Read the model definition and answer for the solid it produces. Units are mm, in the model's axes. A direction names the side the tool comes from. Coordinates: 2 decimals unless noted, no trailing zeros. Order: outer loops, then holes, each group sorted by start corner. A loop starts at its lowest first (then second) coordinate and runs counter-clockwise, first axis right, second up. Notation, with made-up numbers: M -19,79.5 L -15,79.5 A24 ccw -15,108.5 Z; hole C 15,28 d9. An arc over 180 degrees is marked long. Use a Markdown table: item, result. Add a question column.
1) Find the intervals of material crossed by probe 1 along X at (y, z) = (17, -4); probe 2 along X at (y, z) = (4.25, 34.5); probe 3 along Z at (x, y) = (10.5, 22), in increasing order. Write a range as [from, to].
2) Each of these flat-tipped pins is pushed along its axis until it touches: pin 1 Ø6.5 at (y, z) = (9.5, -5) entering from -X; pin 2 Ø4 at (y, z) = (12, 5.5) entering from +X; pin 3 Ø7 at (y, z) = (11, 37.5) entering from -X. Where does it stop, or does it pass through?
3) Find section B-B on z = -4. Write down the section's boundary in (x, y), plus the area to 3 significant figures.
4) Find section D-D on x = 15. Write down the section's boundary in (y, z), plus the area to 3 significant figures.
5) Find section C-C on y = 8.75. Write down the section's boundary in (x, z).
6) The mould has two halves that part along Z. Classify faces 1 (the face through (45, 10, -8)), 2 (the face through (44, 10, 49.85)), 3 (the face through (42.548, 19.57, 45.416)): released by +Z, released by -Z, zero draft, split by the parting line, or undercut.
7) Find section A-A on y = 20.5. Write down the section's boundary in (x, z), plus the area to 3 significant figures.
8) For faces 4 (the face through (54, 10, 32.85)), 5 (the face through (45, 14.5, -4)), 6 (the face through (20, 10, 41.85)), 7 (the face through (40.5, 10, -4)), determine the directions among +Z, -Z, +X, -X, +Y, -Y from which every point of the face is accessible in a straight line to the end or side of a thin tool.
from build123d import *

# Parameters (mm, degrees)
BOSS_EXTRUDE1_DEPTH  = 24.5
SKETCH2_W            = 103
SKETCH2_H            = 41.85
BOSS_EXTRUDE2_DEPTH  = 5
SKETCH3_W            = 46.5
SKETCH3_H            = 27.85
CUT_EXTRUDE1_DEPTH   = 26
SKETCH7_W            = 8
SKETCH7_H            = 3
BOSS_EXTRUDE3_DEPTH  = 8
SKETCH8_R            = 2.5
CUT_EXTRUDE2_DEPTH   = 8
SKETCH9_W            = 8
SKETCH9_H            = 3
BOSS_EXTRUDE4_DEPTH  = 8
SKETCH10_R           = 2.5
CUT_EXTRUDE3_DEPTH   = 8
SKETCH12_W           = 11.5
SKETCH12_H           = 5
CUT_EXTRUDE4_DEPTH   = 8
SKETCH14_W           = 8
SKETCH14_H           = 3
BOSS_EXTRUDE5_DEPTH  = 8
SKETCH15_R           = 2.5
CUT_EXTRUDE5_DEPTH   = 8
SKETCH16_W           = 8
SKETCH16_H           = 29.5
BOSS_EXTRUDE6_DEPTH  = 8
SKETCH17_W           = 14
SKETCH17_H           = 29.5
BOSS_EXTRUDE7_DEPTH  = 8
SKETCH18_R           = 2
CUT_EXTRUDE6_DEPTH   = 10
SKETCH19_W           = 8
SKETCH19_H           = 29.5
BOSS_EXTRUDE8_DEPTH  = 8
SKETCH20_W           = 13
SKETCH20_H           = 13
BOSS_EXTRUDE9_DEPTH  = 88
CUT_EXTRUDE8_DEPTH   = 48
SKETCH23_R           = 2.5
CUT_EXTRUDE9_DEPTH   = 10
SKETCH25_W           = 8
SKETCH25_H           = 3
CUT_EXTRUDE10_DEPTH  = 8
SKETCH27_W           = 8
SKETCH27_H           = 29.5
BOSS_EXTRUDE11_DEPTH = 8
SKETCH28_R           = 2.5
CUT_EXTRUDE12_DEPTH  = 15
SKETCH29_W           = 13
SKETCH29_H           = 13
CUT_EXTRUDE13_DEPTH  = 88
SKETCH30_W           = 14
SKETCH30_H           = 8
CUT_EXTRUDE14_DEPTH  = 147


with BuildPart() as part:
    # Sketch1 → Boss-Extrude1 (new body)
    with BuildSketch(Plane(origin=(0, 0, 0), x_dir=(1, 0, 0), z_dir=(0, 1, 0))):
        Polygon((0, 0), (51.5, 0), (51.5, -5), (5, -5), (5, -36.85), (51.5, -36.85), (51.5, -32.85), (56.5, -32.85), (56.5, -41.85), (0, -41.85), align=None)
    extrude(amount=BOSS_EXTRUDE1_DEPTH)

    # Sketch2 → Boss-Extrude2 (add)
    with BuildSketch(Plane.XZ):
        with Locations((51.5, 20.925)):
            Rectangle(SKETCH2_W, SKETCH2_H)
    extrude(amount=BOSS_EXTRUDE2_DEPTH)

    # Sketch3 → Cut-Extrude1 (cut)
    with BuildSketch(Plane(origin=(0, 0, 0), x_dir=(1, 0, 0), z_dir=(0, 1, 0))):
        with Locations((74.75, -18.925)):
            Rectangle(SKETCH3_W, SKETCH3_H)
    extrude(amount=-CUT_EXTRUDE1_DEPTH, mode=Mode.SUBTRACT)

    # Sketch7 → Boss-Extrude3 (add)
    with BuildSketch(Plane.XY.offset(41.85)):
        with Locations((4, -3.5)):
            Rectangle(SKETCH7_W, SKETCH7_H)
    extrude(amount=BOSS_EXTRUDE3_DEPTH)

    # Sketch8 → Cut-Extrude2 (cut)
    with BuildSketch(Plane(origin=(0, -2, 0), x_dir=(1, 0, 0), z_dir=(0, 1, 0))):
        with Locations(Location((4, -45.85, 0), (0, 0, 270))):
            Circle(SKETCH8_R)
    extrude(amount=-CUT_EXTRUDE2_DEPTH, mode=Mode.SUBTRACT)

    # Sketch9 → Boss-Extrude4 (add)
    with BuildSketch(Plane(origin=(0, 0, 0), x_dir=(-1, 0, 0), z_dir=(0, 0, -1))):
        with Locations((-99, -3.5)):
            Rectangle(SKETCH9_W, SKETCH9_H)
    extrude(amount=BOSS_EXTRUDE4_DEPTH)

    # Sketch10 → Cut-Extrude3 (cut)
    with BuildSketch(Plane(origin=(0, -2, 0), x_dir=(1, 0, 0), z_dir=(0, 1, 0))):
        with Locations(Location((99, 3.996680608, 0), (0, 0, 270))):
            Circle(SKETCH10_R)
    extrude(amount=-CUT_EXTRUDE3_DEPTH, mode=Mode.SUBTRACT)

    # Sketch12 → Cut-Extrude4 (cut)
    with BuildSketch(Plane(origin=(0, 0, 0), x_dir=(1, 0, 0), z_dir=(0, 1, 0))):
        with Locations((89.25, -2.5)):
            Rectangle(SKETCH12_W, SKETCH12_H)
    extrude(amount=-CUT_EXTRUDE4_DEPTH, mode=Mode.SUBTRACT)

    # Sketch14 → Boss-Extrude5 (add)
    with BuildSketch(Plane(origin=(0, 0, 0), x_dir=(-1, 0, 0), z_dir=(0, 0, -1))):
        with Locations((-79.5, -3.5)):
            Rectangle(SKETCH14_W, SKETCH14_H)
    extrude(amount=BOSS_EXTRUDE5_DEPTH)

    # Sketch15 → Cut-Extrude5 (cut)
    with BuildSketch(Plane(origin=(0, -2, 0), x_dir=(1, 0, 0), z_dir=(0, 1, 0))):
        with Locations(Location((79.5, 4, 0), (0, 0, 270))):
            Circle(SKETCH15_R)
    extrude(amount=-CUT_EXTRUDE5_DEPTH, mode=Mode.SUBTRACT)

    # Sketch16 → Boss-Extrude6 (add)
    with BuildSketch(Plane(origin=(0, 0, 0), x_dir=(-1, 0, 0), z_dir=(0, 0, -1))):
        with Locations((-44.5, 9.75)):
            Rectangle(SKETCH16_W, SKETCH16_H)
    extrude(amount=BOSS_EXTRUDE6_DEPTH)

    # Sketch17 → Boss-Extrude7 (add)
    with BuildSketch(Plane.XY.offset(41.85)):
        with Locations((41.5, 9.75)):
            Rectangle(SKETCH17_W, SKETCH17_H)
    extrude(amount=BOSS_EXTRUDE7_DEPTH)

    # Sketch18 → Cut-Extrude6 (cut)
    with BuildSketch(Plane(origin=(0, 24.5, 0), x_dir=(1, 0, 0), z_dir=(0, 1, 0))):
        with Locations(Location((44.5, 4, 0), (0, 0, 270))):
            Circle(SKETCH18_R)
        with Locations(Location((44.5, -45.85, 0), (0, 0, 270))):
            Circle(SKETCH18_R)
    extrude(amount=-CUT_EXTRUDE6_DEPTH, mode=Mode.SUBTRACT)

    # Sketch19 → Boss-Extrude8 (add)
    with BuildSketch(Plane.ZY.offset(-34.5)):
        with Locations((45.85, 9.75)):
            Rectangle(SKETCH19_W, SKETCH19_H)
    extrude(amount=BOSS_EXTRUDE8_DEPTH)

    # Sketch20 → Boss-Extrude9 (add)
    with BuildSketch(Plane(origin=(0, 24.5, 0), x_dir=(1, 0, 0), z_dir=(0, 1, 0))):
        with Locations((33, -43.35)):
            Rectangle(SKETCH20_W, SKETCH20_H)
    extrude(amount=BOSS_EXTRUDE9_DEPTH)

    # Sketch22 → Cut-Extrude8 (cut)
    with BuildSketch(Plane(origin=(0, 0, 0), x_dir=(1, 0, 0), z_dir=(0, 1, 0))):
        Polygon((103, 0), (103, 8), (51.5, 8), (51.5, -32.85), (56.5, -32.85), (98, -32.85), (98, -5), (95, -5), (95, 0), align=None)
        Polygon((103, -41.85), (103, -32.85), (98, -32.85), (56.5, -32.85), (56.5, -41.85), align=None)
        Polygon((103, -32.85), (103, 0), (95, 0), (95, -5), (98, -5), (98, -32.85), align=None)
    extrude(amount=-CUT_EXTRUDE8_DEPTH, mode=Mode.SUBTRACT)

    # Sketch23 → Cut-Extrude9 (cut)
    with BuildSketch(Plane.XZ.offset(5)):
        with Locations(Location((44.5, -4, 0), (0, 0, 270))):
            Circle(SKETCH23_R)
    extrude(amount=-CUT_EXTRUDE9_DEPTH, mode=Mode.SUBTRACT)

    # Sketch25 → Cut-Extrude10 (cut)
    with BuildSketch(Plane.XY.offset(49.85)):
        with Locations((4, -3.5)):
            Rectangle(SKETCH25_W, SKETCH25_H)
    extrude(amount=-CUT_EXTRUDE10_DEPTH, mode=Mode.SUBTRACT)

    # Sketch27 → Boss-Extrude11 (add)
    with BuildSketch(Plane.ZY):
        with Locations((28.85, 9.75)):
            Rectangle(SKETCH27_W, SKETCH27_H)
    extrude(amount=BOSS_EXTRUDE11_DEPTH)

    # Sketch28 → Cut-Extrude12 (cut)
    with BuildSketch(Plane.XZ.offset(5)):
        with Locations(Location((-4, 28.85, 0), (0, 0, 270))):
            Circle(SKETCH28_R)
    extrude(amount=-CUT_EXTRUDE12_DEPTH, mode=Mode.SUBTRACT)

    # Sketch29 → Cut-Extrude13 (cut)
    with BuildSketch(Plane(origin=(0, 112.5, 0), x_dir=(1, 0, 0), z_dir=(0, 1, 0))):
        with Locations((33, -43.35)):
            Rectangle(SKETCH29_W, SKETCH29_H)
    extrude(amount=-CUT_EXTRUDE13_DEPTH, mode=Mode.SUBTRACT)

    # Sketch30 → Cut-Extrude14 (cut)
    with BuildSketch(Plane.XZ.offset(5)):
        with Locations((33.5, 45.85)):
            Rectangle(SKETCH30_W, SKETCH30_H)
    extrude(amount=-CUT_EXTRUDE14_DEPTH, mode=Mode.SUBTRACT)


solid = part.part
Check result:
| question | item | result |
|---|---|---|
| 1 | probe 1 | x = [40.5, 42.5], [46.5, 48.5] |
| 1 | probe 2 | x = [0, 5], [51.5, 56.5] |
| 1 | probe 3 | z = [0, 5], [36.85, 41.85] |
| 2 | pin 1 | stops at x = 40.5 |
| 2 | pin 2 | stops at x = 51.5 |
| 2 | pin 3 | stops at x = 0 |
| 3 | outline | M 40.5,-5 L 42,-5 L 42,5 L 47,5 L 47,-5 L 48.5,-5 L 48.5,24.5 L 46.5,24.5 L 46.5,14.5 L 42.5,14.5 L 42.5,24.5 L 40.5,24.5 Z |
| 3 | area | 146 mm2 |
| 4 | outline | M -5,0 L 24.5,0 L 24.5,5 L 0,5 L 0,36.85 L 24.5,36.85 L 24.5,41.85 L -5,41.85 Z |
| 4 | area | 454 mm2 |
| 5 | outline | M -8,24.85 L 0,24.85 L 0,0 L 40.5,0 L 40.5,-8 L 48.5,-8 L 48.5,0 L 51.5,0 L 51.5,5 L 5,5 L 5,36.85 L 51.5,36.85 L 51.5,32.85 L 56.5,32.85 L 56.5,41.85 L 48.5,41.85 L 48.5,49.85 L 40.5,49.85 L 40.5,41.85 L 0,41.85 L 0,32.85 L -8,32.85 Z; hole C -4,28.85 d5 |
| 6 | face 1 | released by -Z |
| 6 | face 2 | released by +Z |
| 6 | face 3 | undercut |
| 7 | outline | M -8,24.85 L 0,24.85 L 0,0 L 40.5,0 L 40.5,-8 L 48.5,-8 L 48.5,0 L 51.5,0 L 51.5,5 L 5,5 L 5,36.85 L 51.5,36.85 L 51.5,32.85 L 56.5,32.85 L 56.5,41.85 L 48.5,41.85 L 48.5,49.85 L 40.5,49.85 L 40.5,41.85 L 0,41.85 L 0,32.85 L -8,32.85 Z; hole C 44.5,-4 d4; hole C 44.5,45.85 d4 |
| 7 | area | 886 mm2 |
| 8 | face 4 | -Z, +X, +Y, -Y |
| 8 | face 5 | +Y |
| 8 | face 6 | +Z, -X, +Y, -Y |
| 8 | face 7 | -Z, -X, +Y, -Y |
